Can you work these out from the model? Positions are in its coordinate system, mm. Round coordinates to 2 decimals unless told otherwise and drop trailing zeros. Order: outer loops, then holes, each group sorted by start corner. A loop starts at its lowest first (then second) coordinate and runs counter-clockwise, first axis right, second up. Notation, with made-up numbers: M -0.5,58.25 L 49.5,58.25 A11 ccw 49.5,76.25 Z; hole C 3.5,52 d3. An arc over 180 degrees is marked long. Answer as a JSON object with one key per item and string values. Group by question number.
from build123d import *

# Parameters (mm, degrees)
BOSS_EXTRUDE1_DEPTH = 257
BOSS_EXTRUDE1_TAPER = 0.2


with BuildPart() as part:
    # Sketch1 → Boss-Extrude1 (new body)
    with BuildSketch(Plane.XY):
        with BuildLine():
            Line((-805.959430903, -1279.437202161), (-805.959430903, -1277.237202161))
            ThreePointArc((-805.959430903, -1277.237202161), (-806.398770731, -1276.176541989), (-807.459430903, -1275.737202161))
            Line((-807.459430903, -1275.737202161), (-811.259430903, -1275.737202161))
            ThreePointArc((-811.259430903, -1275.737202161), (-812.320091075, -1276.176541989), (-812.759430903, -1277.237202161))
            Line((-812.759430903, -1277.237202161), (-812.759430903, -1279.437202161))
            ThreePointArc((-812.759430903, -1279.437202161), (-812.320091075, -1280.497862332), (-811.259430903, -1280.937202161))
            Line((-811.259430903, -1280.937202161), (-807.459430903, -1280.937202161))
            ThreePointArc((-807.459430903, -1280.937202161), (-806.398770731, -1280.497862332), (-805.959430903, -1279.437202161))
        make_face()
    extrude(amount=BOSS_EXTRUDE1_DEPTH, taper=BOSS_EXTRUDE1_TAPER)


solid = part.part
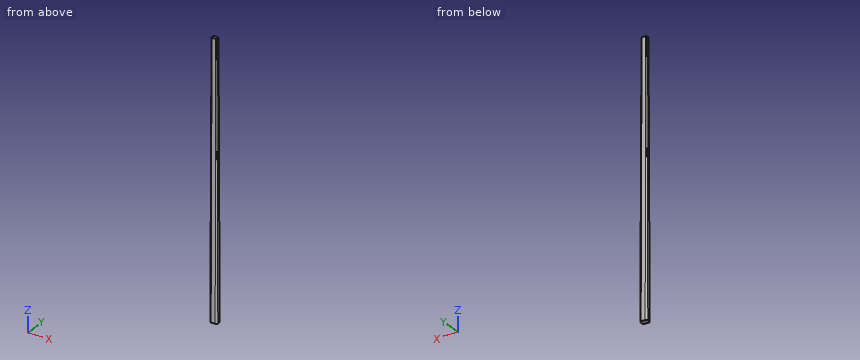
Item 1: I need wall thicknesses on line 1 (Y direction, x = -807.75, z = 11); line 2 (X direction, y = -1280.3, z = 121); line 3 (Y direction, x = -808, z = 231.5). Which ranges of each line are inside material? Lowest first, please.
Item 2: Suppose I cut it at A-A, the plane z = 176. Write out the boundary of the cut face in (x, y).
Item 3: I'm going to push flat-ended pins straight in: pin 1 Ø3 at (x, z) = (-811.5, 170) entering from -Y; pin 2 Ø1 at (y, z) = (-1280.5, 176.5) entering from -X; pin 3 Ø1 at (y, z) = (-1278, 215.5) entering from -X. Where does each tip first touch, or does it pass through?
Item 4: Suppose I cut it at C-C, the plane z = 48. Write out the boundary of the cut face in (x, y).
Item 5: Suppose I cut it at B-B, the plane x = -809.5. Write out the boundary of the cut face in (y, z), and give its area (3 significant figures).
Computed:
{
 "1": {"line 1": "y = -1280.9 to -1275.78", "line 2": "x = -811.91 to -806.81", "line 3": "y = -1280.13 to -1276.55"},
 "2": {"outline": "M -812.15,-1279.44 A0.89 ccw -811.26,-1280.32 L -807.46,-1280.32 A0.89 ccw -806.57,-1279.44 L -806.57,-1277.24 A0.89 ccw -807.46,-1276.35 L -811.26,-1276.35 A0.89 ccw -812.15,-1277.24 Z"},
 "3": {"pin 1": "stops at y = -1280.35", "pin 2": "stops at x = -811.94", "pin 3": "stops at x = -812.01"},
 "4": {"outline": "M -812.59,-1279.44 A1.33 ccw -811.26,-1280.77 L -807.46,-1280.77 A1.33 ccw -806.13,-1279.44 L -806.13,-1277.24 A1.33 ccw -807.46,-1275.9 L -811.26,-1275.9 A1.33 ccw -812.59,-1277.24 Z"},
 "5": {"outline": "M -1280.94,0 L -1275.74,0 L -1276.63,257 L -1280.04,257 Z", "area": "1,110 mm^2"}
}
